Job drawing, mm, ordinate dimensions from the low corner. One solid piece. A direction names the side the tool comes from. Round coordinates to 2 decimals unless told otherwise and drop trailing zeros. Loops run counter-clockwise (first coordinate to the right, second up) from the corner with the lowest first, then second, coordinate; pieces in that order, holes last.
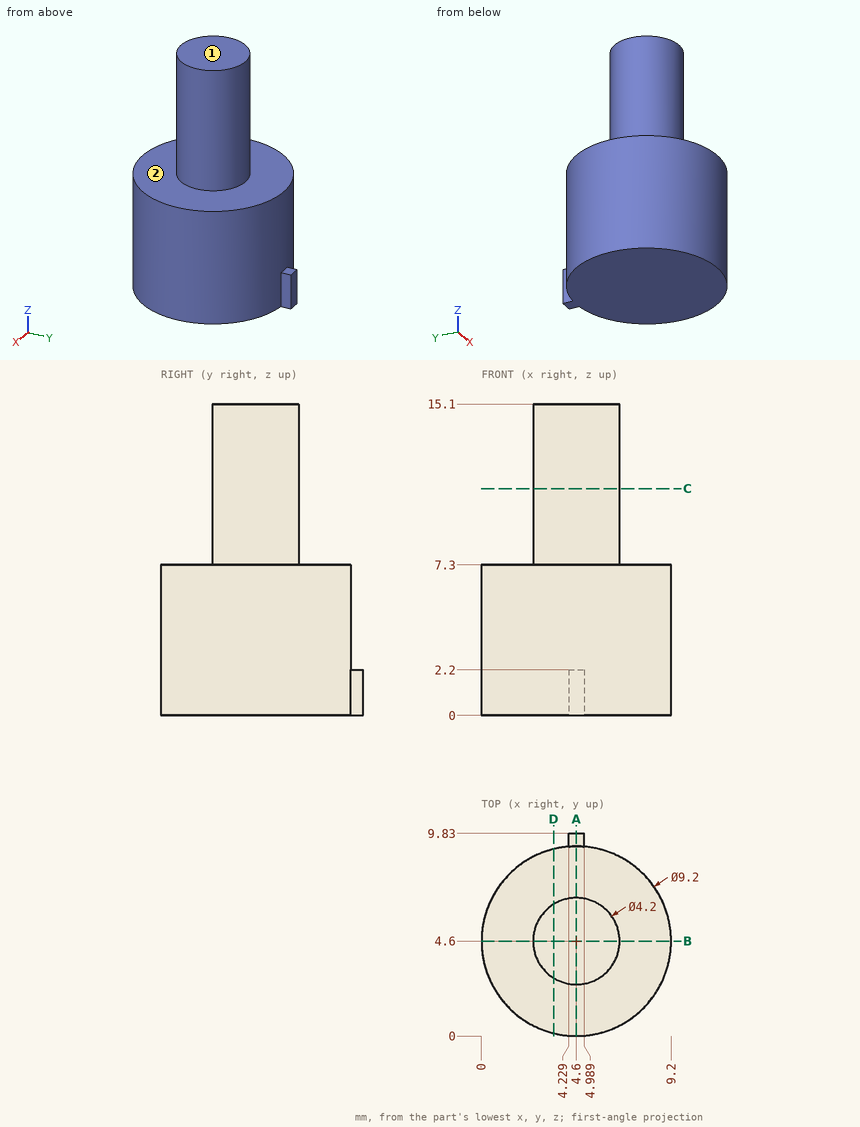
Item 1: Probe line 1 (Z direction, x = 3.5, y = 8); line 2 (Y direction, x = 4.5, z = 6.25). List the from-to ranges inside material, lowest first.
Answers follow:
line 1: z = 0 to 7.3
line 2: y = 0 to 9.2
Item 2: Cut at C-C, the plane z = 11. Give the cut face in (x, y).
Answers follow:
outline: circle Ø4.2 at (4.6, 4.6)
Item 3: 3-axis set-ups, long thin cutter, end or side, ignore diameter. For the marked faces 1 and 2: which of +Z, -Z, +X, -X, +Y, -Y reach the whole face in a straight line?
Answers follow:
face 1: +Z, +X, -X, +Y, -Y
face 2: +Z
Item 4: Cut at B-B, the plane y = 4.6. Give the cut face in (x, z).
Answers follow:
outline: (0, 0) - (9.2, 0) - (9.2, 7.3) - (6.7, 7.3) - (6.7, 15.1) - (2.5, 15.1) - (2.5, 7.3) - (0, 7.3) - close
Item 5: Cut at D-D, the plane x = 3.5. Give the cut face in (y, z).
Answers follow:
outline: (0.13, 0) - (9.07, 0) - (9.07, 7.3) - (6.39, 7.3) - (6.39, 15.1) - (2.81, 15.1) - (2.81, 7.3) - (0.13, 7.3) - close
Item 6: Cut at A-A, the plane x = 4.6. Give the cut face in (y, z), plus the area to 3 significant figures.
Answers follow:
outline: (0, 0) - (9.83, 0) - (9.83, 2.2) - (9.2, 2.2) - (9.2, 7.3) - (6.7, 7.3) - (6.7, 15.1) - (2.5, 15.1) - (2.5, 7.3) - (0, 7.3) - close
area: 101 mm2
Item 7: Flat gauge pins, fed straight in: P1, Ø2, axis at x = 1, z = 7, coming from the +Y side (1 decimal); P2, Ø0.7, axis at x = 5, y = 9.5, coming from the +Z side; P3, Ø4, axis at y = 1, z = 4, coming from the +X side. Where does each tip first touch, or does it go through?
Answers follow:
P1: stops at y = 8.4
P2: stops at z = 7.3
P3: stops at x = 8.91
